For this review, take the finished solid that the model builds, in its own axes (mm). A direction names the side the tool comes from. Round coordinates to 2 decimals unless told otherwise and drop trailing zeros. Write each loop counter-clockwise with the first axis right and the second up, starting at its lowest first coordinate (ties: lowest second). Pieces come first, ordered by that corner, then holes. Notation, with made-up numbers: M 53,7 L 79,7 A14 cw 79,34 Z; hole C 0.5,36.25 d10. An arc over 180 degrees is marked long. Answer in a Markdown table with one row per item.
```python
from build123d import *

# Parameters (mm, degrees)
ESQUISSE1_R        = 1.05
ESQUISSE1_R_2      = 1.3
ESQUISSE1_R_3      = 0.625
ESQUISSE1_R_4      = 0.9
ESQUISSE1_R_5      = 4
BOSS_EXTRU_1_DEPTH = 2


with BuildPart() as part:
    # Esquisse1 → Boss.-Extru.1 (new body)
    with BuildSketch(Plane.XY):
        with BuildLine():
            Line((-145, 15), (-149, 15))
            Line((-149, 15), (-149, -1))
            Line((-149, -1), (-145, -1))
            Line((-145, -1), (-145, -2))
            ThreePointArc((-145, -2), (-137.928932188, -4.928932188), (-135, -12))
            Line((-135, -12), (-135, -13))
            Line((-135, -13), (-127.168338795, -13))
            Line((-127.168338795, -13), (-124.67428839, -3.468568753))
            ThreePointArc((-124.67428839, -3.468568753), (-121.110879132, 1.915627343), (-115, 4))
            Line((-115, 4), (-92.916549028, 4))
            ThreePointArc((-92.916549028, 4), (-86.162816659, 0.304952282), (-84, -7.083450972))
            Line((-84, -7.083450972), (-84, -20))
            Line((-84, -20), (-33.5, -20))
            Line((-33.5, -20), (-33.5, -3))
            Line((-33.5, -3), (-20.5, -3))
            Line((-20.5, -3), (-20.5, -20))
            Line((-20.5, -20), (17.5, -20))
            Line((17.5, -20), (17.5, -3))
            Line((17.5, -3), (30.5, -3))
            Line((30.5, -3), (30.5, -20))
            Line((30.5, -20), (70.5, -20))
            Line((70.5, -20), (70.5, -3))
            Line((70.5, -3), (83.5, -3))
            Line((83.5, -3), (83.5, -20))
            Line((83.5, -20), (113, -20))
            Line((113, -20), (113, -17))
            ThreePointArc((113, -17), (113.878679656, -14.878679656), (116, -14))
            Line((116, -14), (134.596227596, -14))
            Line((134.596227596, -14), (135.202041029, -10))
            ThreePointArc((135.202041029, -10), (138.67544468, -4.254033308), (145, -2))
            Line((145, -2), (145, -1))
            Line((145, -1), (149, -1))
            Line((149, -1), (149, 15))
            Line((149, 15), (145, 15))
            Line((145, 15), (145, 16))
            Line((145, 16), (-9.00367652, 16))
            ThreePointArc((-9.00367652, 16), (-13.00367652, 12), (-17.00367652, 16))
            Line((-17.00367652, 16), (-38, 16))
            ThreePointArc((-38, 16), (-40.121320344, 16.878679656), (-41, 19))
            Line((-41, 19), (-41, 20))
            Line((-41, 20), (-135, 20))
            Line((-135, 20), (-135, 16))
            Line((-135, 16), (-145, 16))
            Line((-145, 16), (-145, 15))
        make_face()
        with Locations((-79, -16)):
            Circle(ESQUISSE1_R, mode=Mode.SUBTRACT)
        with Locations((-59, -16)):
            Circle(ESQUISSE1_R, mode=Mode.SUBTRACT)
        with Locations((-1.5, -13)):
            Circle(ESQUISSE1_R_2, mode=Mode.SUBTRACT)
        with Locations((-133, -10)):
            Circle(ESQUISSE1_R_3, mode=Mode.SUBTRACT)
        with Locations((-129, -10)):
            Circle(ESQUISSE1_R_3, mode=Mode.SUBTRACT)
        with Locations((109, -14)):
            Circle(ESQUISSE1_R_2, mode=Mode.SUBTRACT)
        with Locations((50.5, -10)):
            Circle(ESQUISSE1_R_4, mode=Mode.SUBTRACT)
        with BuildLine():
            ThreePointArc((103.5, 3), (104.560660172, 2.560660172), (105, 1.5))
            Line((105, 1.5), (105, -6.5))
            ThreePointArc((105, -6.5), (104.560660172, -7.560660172), (103.5, -8))
            Line((103.5, -8), (93.5, -8))
            ThreePointArc((93.5, -8), (92.439339828, -7.560660172), (92, -6.5))
            Line((92, -6.5), (92, 1.5))
            ThreePointArc((92, 1.5), (92.439339828, 2.560660172), (93.5, 3))
            Line((93.5, 3), (103.5, 3))
        make_face(mode=Mode.SUBTRACT)
        with BuildLine():
            Line((114.5, 3), (124.5, 3))
            ThreePointArc((124.5, 3), (125.560660172, 2.560660172), (126, 1.5))
            Line((126, 1.5), (126, -6.5))
            ThreePointArc((126, -6.5), (125.560660172, -7.560660172), (124.5, -8))
            Line((124.5, -8), (114.5, -8))
            ThreePointArc((114.5, -8), (113.439339828, -7.560660172), (113, -6.5))
            Line((113, -6.5), (113, 1.5))
            ThreePointArc((113, 1.5), (113.439339828, 2.560660172), (114.5, 3))
        make_face(mode=Mode.SUBTRACT)
        with Locations((-79, 1.5)):
            Circle(ESQUISSE1_R, mode=Mode.SUBTRACT)
        with Locations((-146.5, 7)):
            Circle(ESQUISSE1_R, mode=Mode.SUBTRACT)
        with Locations((-132, 8)):
            Circle(ESQUISSE1_R_4, mode=Mode.SUBTRACT)
        with Locations((-112, 8)):
            Circle(ESQUISSE1_R_4, mode=Mode.SUBTRACT)
        with Locations((-69, 1.5)):
            Circle(ESQUISSE1_R_5, mode=Mode.SUBTRACT)
        with Locations((-59, 1.5)):
            Circle(ESQUISSE1_R, mode=Mode.SUBTRACT)
        with Locations((-49, 8)):
            Circle(ESQUISSE1_R_4, mode=Mode.SUBTRACT)
        with Locations((-132, 15)):
            Circle(ESQUISSE1_R_4, mode=Mode.SUBTRACT)
        with Locations((-112, 15)):
            Circle(ESQUISSE1_R_4, mode=Mode.SUBTRACT)
        with Locations((-49, 15)):
            Circle(ESQUISSE1_R_4, mode=Mode.SUBTRACT)
        with Locations((50.5, 2)):
            Circle(ESQUISSE1_R_4, mode=Mode.SUBTRACT)
        with Locations((46, 8)):
            Circle(ESQUISSE1_R_3, mode=Mode.SUBTRACT)
        with Locations((146.5, 7)):
            Circle(ESQUISSE1_R, mode=Mode.SUBTRACT)
        with Locations((20, 11)):
            Circle(ESQUISSE1_R_3, mode=Mode.SUBTRACT)
        with Locations((28, 11)):
            Circle(ESQUISSE1_R_3, mode=Mode.SUBTRACT)
        with Locations((2.5, 13)):
            Circle(ESQUISSE1_R_3, mode=Mode.SUBTRACT)
        with Locations((63, 13)):
            Circle(ESQUISSE1_R_4, mode=Mode.SUBTRACT)
        with Locations((46, 15)):
            Circle(ESQUISSE1_R_3, mode=Mode.SUBTRACT)
    extrude(amount=BOSS_EXTRU_1_DEPTH)


solid = part.part
```
Q1. For probe 1 along Y at (x, z) = (-49, 1.2); probe 2 along Y at (x, z) = (-132, 1); probe 3 along X at (y, z) = (-16.5, 0.85), list the stretches that pass through material, from the lowest coordinate up.
Found:
| item | result |
|---|---|
| probe 1 | -20 to 7.1, 8.9 to 14.1, 15.9 to 20 |
| probe 2 | -13 to 7.1, 8.9 to 14.1, 15.9 to 20 |
| probe 3 | -84 to -79.92, -78.08 to -59.92, -58.08 to -33.5, -20.5 to 17.5, 30.5 to 70.5, 83.5 to 113.04 |
Q2. Take a section at B-B (z = 0.5). State how many separate pieces and enclosed holes the cut face has, then the cut area to 3 significant figures.
Found:
| item | result |
|---|---|
| separate pieces | 1 |
| enclosed holes | 27 |
| area | 8,390 mm² |
Q3. Mouldability with a two-part tool opening along X and no side actions: class faces 3 (the face through (-2, 0, 2)), 4 (the face through (-86.23, 0.39, 0.99)), 5 (the face through (-138.01, -4.85, 0.99)) as +X half, -X half, draft (parallel to the pull), parting line (faces both ways), or undercut.
Found:
| item | result |
|---|---|
| face 3 | draft |
| face 4 | undercut |
| face 5 | -X half |
Q4. Take a section at A-A (x = -69). State the section outline as (y, z) points.
Found:
| item | result |
|---|---|
| outline | M -20,0 L -2.5,0 L -2.5,2 L -20,2 Z; M 5.5,0 L 20,0 L 20,2 L 5.5,2 Z |
Q5. Machinability: for faces 1 (the face through (-65.305, -0.032, 0.986)), 2 (the face through (-121, 2, 1)), which of the approach directions +Z, -Z, +X, -X, +Y, -Y give a long, thin tool a straight path to every point of the face, cutting with its end or side? Answer none if there is none.
Found:
| item | result |
|---|---|
| face 1 | +Z, -Z |
| face 2 | +Z, -Z, -Y |
Q6. Take a section at C-C (x = 67.5). State the section outline as (y, z) points.
Found:
| item | result |
|---|---|
| outline | M -20,0 L 16,0 L 16,2 L -20,2 Z |
Q7. Insertion check: P1, Ø0.6, axis at x = -141.5, z = 1.5, coming from the +Y side; P2, Ø5, axis at x = 110.5, y = 9, coming from the -Z side; P3, Ø0.6, axis at x = 78.5, z = 0.5, coming from the -Y side. Each pin has a flat end and moves straight along its axis. Give the tip position at first contact, or say it passes through.
Found:
| item | result |
|---|---|
| P1 | y = 16 |
| P2 | z = 0 |
| P3 | y = -3 |
